Input: dimensioned drawing with shaded views. Units: mm. Origin: part minimum x, y, z. Round coordinates to 2 decimals unless told otherwise and drop trailing zeros. Write each loop counter-clockwise with the first axis right and the second up, starting at its lowest first coordinate (ties: lowest second). Pieces come first, ordered by that corner, then holes. Notation, with made-up numbers: M 54,6.25 L 97,6.25 A10 ccw 97,15.25 Z; hole C 31.5,77.25 d2. An arc over 180 degrees is marked long. Answer in a Markdown table with one row per item. Add a question column.
Item 1: Cut plane A-A on y = 7.5. Return loops of the section in (x, z).
Item 2: Material intervals for probe 1 along X at (y, z) = (7.5, 1.6); probe 2 along Y at (x, z) = (5, 0.9); probe 3 along X at (y, z) = (90, 0.75), sorted ascending.
Item 3: Cut plane B-B on x = 14.5. Return loops of the section in (y, z), and give its area (3 significant figures).
Item 4: Contact query for a flat-ended pin moving along its axis: pin 1 (2.5 mm diameter, centred on x = 15, y = 112.5, fed in from +Z). Output: stop coordinate, or through.
Item 5: Cut plane D-D on z = 1.15. Return loops of the section in (x, y), and give its area (3 significant figures).
Item 6: Cut plane C-C on y = 100. Return loops of the section in (x, z).
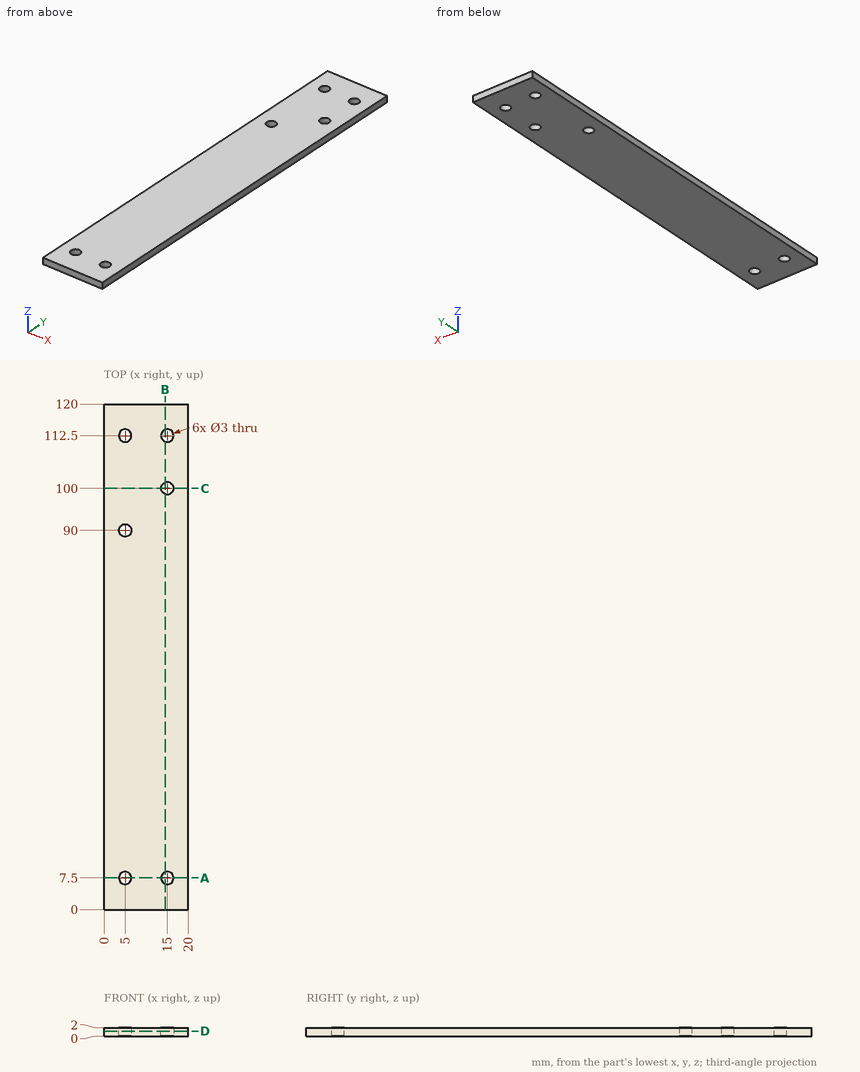
Results below:
| question | item | result |
|---|---|---|
| 1 | outline | M 0,0 L 3.5,0 L 3.5,2 L 0,2 Z; M 6.5,0 L 13.5,0 L 13.5,2 L 6.5,2 Z; M 16.5,0 L 20,0 L 20,2 L 16.5,2 Z |
| 2 | probe 1 | 0 to 3.5, 6.5 to 13.5, 16.5 to 20 |
| 2 | probe 2 | 0 to 6, 9 to 88.5, 91.5 to 111, 114 to 120 |
| 2 | probe 3 | 0 to 3.5, 6.5 to 20 |
| 3 | outline | M 0,0 L 6.09,0 L 6.09,2 L 0,2 Z; M 8.91,0 L 98.59,0 L 98.59,2 L 8.91,2 Z; M 101.41,0 L 111.09,0 L 111.09,2 L 101.41,2 Z; M 113.91,0 L 120,0 L 120,2 L 113.91,2 Z |
| 3 | area | 223 mm2 |
| 4 | pin 1 | through |
| 5 | outline | M 0,0 L 20,0 L 20,120 L 0,120 Z; hole C 5,7.5 d3; hole C 5,90 d3; hole C 5,112.5 d3; hole C 15,7.5 d3; hole C 15,100 d3; hole C 15,112.5 d3 |
| 5 | area | 2,360 mm2 |
| 6 | outline | M 0,0 L 13.5,0 L 13.5,2 L 0,2 Z; M 16.5,0 L 20,0 L 20,2 L 16.5,2 Z |
